```python
from build123d import *

# Parameters (mm, degrees)
EXTRUDE1_DEPTH          = 3.25
SKETCH13_R              = 4
BOSS_EXTRUDE1_DEPTH     = 6.5
SKETCH7_OUTSIDE_W       = 107.168
SKETCH7_OUTSIDE_H       = 109.18
SKETCH7_OUTSIDE_R       = 6.5
EXTRUDE2_DEPTH          = 25.4
EXTRUDE2_DRAFT          = -60
MIRROR2_COPY_1_SKETCH_W = 107.168
MIRROR2_COPY_1_SKETCH_H = 109.18
MIRROR2_COPY_1_SKETCH_R = 6.5
MIRROR2_COPY_1_DEPTH    = 25.4
MIRROR2_COPY_1_DRAFT    = -60


with BuildPart() as part:
    # Sketch1 → Extrude1 (new, symmetric)
    with BuildSketch(Plane.XY):
        Polygon((-6.5, 3.75277675), (-6.5, -3.75277675), (0, -7.505553499), (6.5, -3.75277675), (6.5, 3.75277675), (0, 7.505553499), align=None)
    extrude(amount=EXTRUDE1_DEPTH, both=True)

    # Cut-Extrude2 cone 1 section (through the dimple's axis) → Cut-Extrude2 (revolve, cut)
    with BuildSketch(Plane(origin=(0, 0, 3.25), x_dir=(0, -1, 0), z_dir=(1, 0, 0))):
        Polygon((0, 0), (4, 0), (0, 4), align=None)
    revolve(axis=Axis((0, 0, 3.25), (0, 0, -1)), mode=Mode.SUBTRACT)

    # Cut-Extrude3 cone 1 section (through the dimple's axis) → Cut-Extrude3 (revolve, cut)
    with BuildSketch(Plane(origin=(0, 0, -3.25), x_dir=(0, 1, 0), z_dir=(1, 0, 0))):
        Polygon((0, 0), (4, 0), (0, 4), align=None)
    revolve(axis=Axis((0, 0, -3.25), (0, 0, 1)), mode=Mode.SUBTRACT)


with BuildPart() as body_2:
    # Sketch13 → Boss-Extrude1 (new body)
    with BuildSketch(Plane(origin=(0, 0, -3.25), x_dir=(-1, 0, 0), z_dir=(0, 0, -1))):
        Circle(SKETCH13_R)
    extrude(amount=-BOSS_EXTRUDE1_DEPTH)


with BuildPart() as part_1:
    add(part.part)

    # Combine1: cut body 2
    add(body_2.part, mode=Mode.SUBTRACT)


with BuildPart() as extrude2_tool:
    # Sketch7 outside → Extrude2 (with draft: the straight prism first)
    with BuildSketch(Plane.XY.offset(3.25)):
        Rectangle(SKETCH7_OUTSIDE_W, SKETCH7_OUTSIDE_H)
        Circle(SKETCH7_OUTSIDE_R, mode=Mode.SUBTRACT)
    extrude(amount=-EXTRUDE2_DEPTH)
    # Extrude2: the draft: its side faces are tilted about the plane it starts from
    extrude2_sides = [extrude2_tool.faces().sort_by_distance(p)[0] for p in [
        (0, -54.59, -9.45),
        (53.584, 0, -9.45),
        (0, 54.59, -9.45),
        (-53.584, 0, -9.45),
        (-6.5, 0, -9.45),
    ]]
    draft(extrude2_sides, Plane.XY.offset(3.25), EXTRUDE2_DRAFT)


with BuildPart() as part_2:
    add(part_1.part)

    # Extrude2: cut by extrude2_tool
    add(extrude2_tool.part, mode=Mode.SUBTRACT)


with BuildPart() as mirror2_copy_1_tool:
    # Mirror2 copy 1 sketch → Mirror2 copy 1 (with draft: the straight prism first)
    with BuildSketch(Plane(origin=(0, 0, -3.25), x_dir=(1, 0, 0), z_dir=(0, 0, -1))):
        Rectangle(MIRROR2_COPY_1_SKETCH_W, MIRROR2_COPY_1_SKETCH_H)
        Circle(MIRROR2_COPY_1_SKETCH_R, mode=Mode.SUBTRACT)
    extrude(amount=-MIRROR2_COPY_1_DEPTH)
    # Mirror2 copy 1: the draft: its side faces are tilted about the plane it starts from
    mirror2_copy_1_sides = [mirror2_copy_1_tool.faces().sort_by_distance(p)[0] for p in [
        (0, -54.59, 9.45),
        (53.584, 0, 9.45),
        (0, 54.59, 9.45),
        (-53.584, 0, 9.45),
        (-6.5, 0, 9.45),
    ]]
    draft(mirror2_copy_1_sides, Plane(origin=(0, 0, -3.25), x_dir=(1, 0, 0), z_dir=(0, 0, -1)), MIRROR2_COPY_1_DRAFT)


with BuildPart() as part_3:
    add(part_2.part)

    # Mirror2 copy 1: cut by mirror2_copy_1_tool
    add(mirror2_copy_1_tool.part, mode=Mode.SUBTRACT)


solid = part_3.part
```
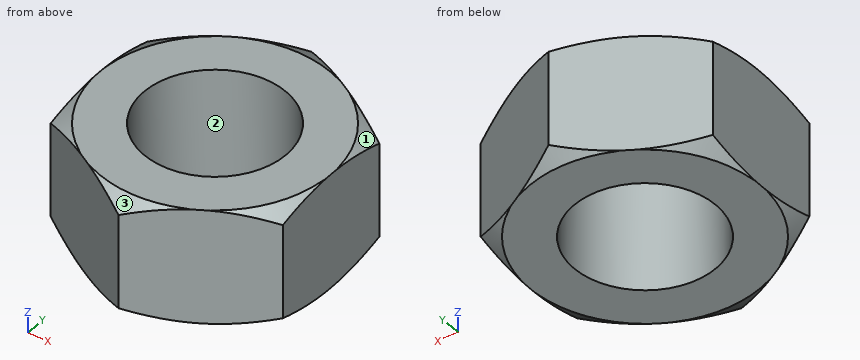
The model under review builds one solid part; all positions refer to its coordinate system, in mm. Face numbers are marked on the shaded views. Round coordinates to 2 decimals unless told otherwise and drop trailing zeros. Write each loop counter-clockwise with the first axis right and the second up, starting at its lowest first coordinate (ties: lowest second). Pieces come first, ordered by that corner, then holes.
(1) Insertion check: pin 1 (1.5 mm diameter, centred on x = -0.5, z = 0.5, fed in from +Y); pin 2 (1 mm diameter, centred on y = 4.5, z = 0.5, fed in from -X). Each pin has a flat end and moves straight along its axis. Give the tip position at first contact, or say it passes through.
(2) Wall thickness on L1, parallel to X at y = 0, z = 0; L2, parallel to Y at x = -2.5, z = 1.5; L3, parallel to Y at x = -3, z = -1.25: over which ranges is each line inside the solid? List them lowest first.
(3) We need section A-A on z = 2.5. Give the boundary of the cut face in (x, y), and give its area (3 significant figures).
(4) Mouldability with a two-part tool opening along Y and no side actions: class the marked faces 1, 2 and 3 as +Y half, -Y half, draft (parallel to the pull), parting line (faces both ways), or undercut.
Findings below:
1. pin 1: stops at y = 7.51
1. pin 2: stops at x = -6.07
2. L1: x = -6.5 to -4, 4 to 6.5
2. L2: y = -6.06 to -3.12, 3.12 to 6.06
2. L3: y = -5.77 to -2.65, 2.65 to 5.77
3. outline: (-6.5, -3.75) - (0, -7.51) - (6.5, -3.75) - (6.5, 3.75) - (0, 7.51) - (-6.5, 3.75) - close; hole circle Ø8 at (0, 0)
3. area: 96.1 mm2
4. face 1: +Y half
4. face 2: undercut
4. face 3: -Y half
